from build123d import *

# Parameters (mm, degrees)
SKETCH_1_W          = 54
SKETCH_1_H          = 18
EXTRUDE_1_DEPTH     = 2.5
SKETCH_2_W          = 40
SKETCH_2_H          = 18
EXTRUDE_2_DEPTH     = 28
SKETCH_3_W          = 40
SKETCH_3_H          = 18
EXTRUDE_3_DEPTH     = 6.7
SKETCH_4_R          = 7.5
EXTRUDE_4_DEPTH     = 3.6
SKETCH_5_R          = 3
EXTRUDE_5_DEPTH     = 4.5
SKETCH_6_R          = 2
CUT_EXTRUDE_1_DEPTH = 4.5


with BuildPart() as part:
    # 草图1 → 凸台-拉伸1 (new body)
    with BuildSketch(Plane(origin=(0, 0, 0), x_dir=(1, 0, 0), z_dir=(0, 1, 0))):
        Rectangle(SKETCH_1_W, SKETCH_1_H)
    extrude(amount=EXTRUDE_1_DEPTH)

    # 草图2 → 凸台-拉伸2 (add)
    with BuildSketch(Plane(origin=(0, 2.5, 0), x_dir=(1, 0, 0), z_dir=(0, 1, 0))):
        Rectangle(SKETCH_2_W, SKETCH_2_H)
    extrude(amount=EXTRUDE_2_DEPTH)

    # 草图3 → 凸台-拉伸3 (add)
    with BuildSketch(Plane.XZ):
        Rectangle(SKETCH_3_W, SKETCH_3_H)
    extrude(amount=EXTRUDE_3_DEPTH)

    # 草图4 → 凸台-拉伸4 (add)
    with BuildSketch(Plane.XZ.offset(6.7)):
        with Locations(Location((-10, 0, 0), (0, 0, 90))):
            Circle(SKETCH_4_R)
    extrude(amount=EXTRUDE_4_DEPTH)

    # 草图5 → 凸台-拉伸5 (add)
    with BuildSketch(Plane.XZ.offset(10.3)):
        with Locations(Location((-10, 0, 0), (0, 0, 270))):
            Circle(SKETCH_5_R)
    extrude(amount=EXTRUDE_5_DEPTH)

    # 草图6 → 切除-拉伸1 (cut)
    with BuildSketch(Plane.XZ):
        with Locations(Location((-24.25, 4.75, 0), (0, 0, 270))):
            Circle(SKETCH_6_R)
        with Locations(Location((-24.25, -4.75, 0), (0, 0, 270))):
            Circle(SKETCH_6_R)
        with Locations(Location((24.25, 4.75, 0), (0, 0, 270))):
            Circle(SKETCH_6_R)
        with Locations(Location((24.25, -4.75, 0), (0, 0, 270))):
            Circle(SKETCH_6_R)
    extrude(amount=-CUT_EXTRUDE_1_DEPTH, mode=Mode.SUBTRACT)


solid = part.part
Work out the finished part from the listing and answer in its coordinate system (mm). A direction names the side the tool comes from. Round coordinates to 2 decimals unless told otherwise and drop trailing zeros. Write each loop counter-clockwise with the first axis right and the second up, starting at its lowest first coordinate (ties: lowest second). Pieces come first, ordered by that corner, then holes. Notation, with made-up numbers: (2.25, -29) - (56.25, -29) arc R10 ccw to (56.25, -24) - close; hole circle Ø7 at (5, 21.5). An arc over 180 degrees is marked (long way). Answer in a Markdown table with one row per item. Add a question column.
1. A cutting plane is placed at D-D, the plane y = 22. Determine the outline of the cut face in (x, z), and give its area (3 significant figures).
2. Find the intervals of material crossed by line 1 along X through (y, z) = (1.95, -4.75); line 2 along Y through (x, z) = (-21.5, -2.25); line 3 along Y through (x, z) = (7.5, -0.25), in increasing order. Write a range as from..to.
3. A cutting plane is placed at A-A, the plane x = -24.25. Determine the outline of the cut face in (y, z), and give its area (3 significant figures).
4. The mould has two halves that part along X. Classify faces 5 (the flat face through (-27, 1, 0)), 6 (the cylindrical face through (-24.162, 1.232, -2.752)), 7 (the flat face through (4, -6.7, 0)): +X half, -X half, draft (parallel to the pull), parting line (faces both ways), or undercut.
5. For faces 1 (the flat face through (-24, 2.5, 0)), 2 (the flat face through (20, 16, 0)), 3 (the flat face through (-6.8, -10.3, -0.1)), 4 (the flat face through (23, 0, 0)), determine the directions among +Z, -Z, +X, -X, +Y, -Y from which every point of the face is accessible in a straight line to the end or side of a thin tool.
6. Given pin 1 (5.5 mm diameter, centred on x = 23, z = -2.5, fed in from +Y); pin 2 (3.5 mm diameter, centred on x = 25, z = -2, fed in from -Y); pin 3 (10 mm diameter, centred on y = -9, z = 4.5, fed in from +X), each flat-ended and moving along its own axis, determine where each tip first touches the part or whether it passes through.
7. A cutting plane is placed at C-C, the plane x = -10. Determine the outline of the cut face in (y, z).
8. A cutting plane is placed at B-B, the plane z = 4.75. Determine the outline of the cut face in (x, y), and give its area (3 significant figures).
Worked out:
| question | item | result |
|---|---|---|
| 1 | outline | (-20, -9) - (20, -9) - (20, 9) - (-20, 9) - close |
| 1 | area | 720 mm^2 |
| 2 | line 1 | -27..-26.25, -22.25..22.25, 26.25..27 |
| 2 | line 2 | 0..2.5 |
| 2 | line 3 | -6.7..30.5 |
| 3 | outline | (0, -9) - (2.5, -9) - (2.5, -6.75) - (0, -6.75) - close; (0, -2.75) - (2.5, -2.75) - (2.5, 2.75) - (0, 2.75) - close; (0, 6.75) - (2.5, 6.75) - (2.5, 9) - (0, 9) - close |
| 3 | area | 25.0 mm^2 |
| 4 | face 5 | -X half |
| 4 | face 6 | undercut |
| 4 | face 7 | draft |
| 5 | face 1 | +Z, -Z, -X, +Y |
| 5 | face 2 | +Z, -Z, +X, +Y |
| 5 | face 3 | -Y |
| 5 | face 4 | +Z, -Z, +X, -Y |
| 6 | pin 1 | y = 2.5 |
| 6 | pin 2 | y = 0 |
| 6 | pin 3 | x = 20 |
| 7 | outline | (-14.8, -3) - (-10.3, -3) - (-10.3, -7.5) - (-6.7, -7.5) - (-6.7, -9) - (30.5, -9) - (30.5, 9) - (-6.7, 9) - (-6.7, 7.5) - (-10.3, 7.5) - (-10.3, 3) - (-14.8, 3) - close |
| 8 | outline | (-27, 0) - (-26.25, 0) - (-26.25, 2.5) - (-27, 2.5) - close; (-22.25, 0) - (-20, 0) - (-20, -6.7) - (-15.8, -6.7) - (-15.8, -10.3) - (-4.2, -10.3) - (-4.2, -6.7) - (20, -6.7) - (20, 0) - (22.25, 0) - (22.25, 2.5) - (20, 2.5) - (20, 30.5) - (-20, 30.5) - (-20, 2.5) - (-22.25, 2.5) - close; (26.25, 0) - (27, 0) - (27, 2.5) - (26.25, 2.5) - close |
| 8 | area | 1,540 mm^2 |
